Build history of the part. All positions in model axes, mm. A direction names the side the tool comes from. Give positions to 0.01 mm unless a question says otherwise; leave off trailing zeros. Order: outer loops, then holes, each group sorted by start corner. A loop starts at its lowest first (then second) coordinate and runs counter-clockwise, first axis right, second up. Notation, with made-up numbers: (84.25, 46) - (101.25, 46) arc R24 ccw to (101.25, 57) - close; hole circle Ø10 at (17.25, 60). An arc over 180 degrees is marked (long way). Use a Markdown table: item, result. Add a question column.
(1) Slice it at B-B (z = 94). Write the cut outline in (x, y).
(2) Flat gauge pin, fed straight in: pin 1 (2.5 mm diameter, centred on y = 0, z = 243.79, fed in from -X). Where does the tip first touch, or does it go through?
(3) Mould opens along X. For faces 1 (the face through (0, -7, 253)), 2 (the face through (-7.5, 0, 125)), 3 (the face through (7.5, 0, 125)), 4 (the face through (0.09, -6.74, 1.95)) say: +X half, -X half, draft (parallel to the pull), parting line (faces both ways), or undercut.
(4) Wall check: line 1 (X direction, y = 2.5, z = 176.5); line 2 (X direction, y = -6.95, z = 112). Give the ranges that are in metal, low to high.
(5) Slice it at A-A (z = 53). Write the cut outline in (x, y), then the cut area to 3 significant figures.
(6) Which spindle directions (+Z, -Z, +X, -X, +Y, -Y) get a long thin tool onto all of the face, cutting with end or side? Do faces 5 (the face through (-6.74, 0.09, 55.05)), 6 (the face through (6, 0, 125)). Say none if no direction does.
from build123d import *

# Parameters (mm, degrees)
SKETCH_1_W          = 15
SKETCH_1_H          = 15
SKETCH_1_W_2        = 12
SKETCH_1_H_2        = 12
EXTRUDE_1_DEPTH     = 375
SKETCH_3_R          = 2.05
CUT_EXTRUDE_2_DEPTH = 21
SKETCH_4_R          = 2.05
CUT_EXTRUDE_3_DEPTH = 25
SKETCH_6_R          = 2
CUT_EXTRUDE_5_DEPTH = 75
SKETCH_7_R          = 2
CUT_EXTRUDE_6_DEPTH = 376.374812687
SKETCH_8_W          = 122
SKETCH_8_H          = 15
CUT_EXTRUDE_7_DEPTH = 376.374812687
SKETCH_9_R          = 1.5
CUT_EXTRUDE_8_DEPTH = 254.55522081


with BuildPart() as part:
    # 草图1 → 凸台-拉伸1 (new body)
    with BuildSketch(Plane.XY):
        Rectangle(SKETCH_1_W, SKETCH_1_H)
        Rectangle(SKETCH_1_W_2, SKETCH_1_H_2, mode=Mode.SUBTRACT)
    extrude(amount=EXTRUDE_1_DEPTH)

    # 草图3 → 切除-拉伸2 (cut)
    with BuildSketch(Plane(origin=(0, 7.5, 0), x_dir=(1, 0, 0), z_dir=(0, 1, 0))):
        with Locations(Location((0, -4, 0), (0, 0, 270))):
            Circle(SKETCH_3_R)
        with Locations(Location((0, -12, 0), (0, 0, 270))):
            Circle(SKETCH_3_R)
    extrude(amount=-CUT_EXTRUDE_2_DEPTH, mode=Mode.SUBTRACT)

    # 草图4 → 切除-拉伸3 (cut)
    with BuildSketch(Plane(origin=(7.5, 0, 0), x_dir=(0, 0, -1), z_dir=(1, 0, 0))):
        with Locations((-23, 0)):
            Circle(SKETCH_4_R)
        with Locations((-53, 0)):
            Circle(SKETCH_4_R)
    extrude(amount=-CUT_EXTRUDE_3_DEPTH, mode=Mode.SUBTRACT)

    # 草图6 → 切除-拉伸5 (cut)
    with BuildSketch(Plane(origin=(0, 7.5, 0), x_dir=(1, 0, 0), z_dir=(0, 1, 0))):
        with Locations(Location((0, -335, 0), (0, 0, 270))):
            Circle(SKETCH_6_R)
        with Locations(Location((0, -350, 0), (0, 0, 270))):
            Circle(SKETCH_6_R)
    extrude(amount=-CUT_EXTRUDE_5_DEPTH, mode=Mode.SUBTRACT)

    # 草图7 → 切除-拉伸6 (cut, through all)
    with BuildSketch(Plane(origin=(7.5, 0, 0), x_dir=(0, 0, -1), z_dir=(1, 0, 0))):
        with Locations((-253.786796565, 0)):
            Circle(SKETCH_7_R)
        with Locations((-243.786796565, 0)):
            Circle(SKETCH_7_R)
    extrude(amount=-CUT_EXTRUDE_6_DEPTH, mode=Mode.SUBTRACT)

    # 草图8 → 切除-拉伸7 (cut, through all)
    with BuildSketch(Plane(origin=(7.5, 0, 0), x_dir=(0, 0, -1), z_dir=(1, 0, 0))):
        with Locations((-314, 0)):
            Rectangle(SKETCH_8_W, SKETCH_8_H)
    extrude(amount=-CUT_EXTRUDE_7_DEPTH, mode=Mode.SUBTRACT)

    # 草图9 → 切除-拉伸8 (cut, through all)
    with BuildSketch(Plane(origin=(0, 7.5, 0), x_dir=(1, 0, 0), z_dir=(0, 1, 0))):
        with Locations(Location((0, -218, 0), (0, 0, 270))):
            Circle(SKETCH_9_R)
        with Locations(Location((0, -208, 0), (0, 0, 270))):
            Circle(SKETCH_9_R)
        with Locations(Location((0, -170, 0), (0, 0, 270))):
            Circle(SKETCH_9_R)
        with Locations(Location((0, -160, 0), (0, 0, 270))):
            Circle(SKETCH_9_R)
        with Locations(Location((0, -122, 0), (0, 0, 270))):
            Circle(SKETCH_9_R)
        with Locations(Location((0, -112, 0), (0, 0, 270))):
            Circle(SKETCH_9_R)
        with Locations(Location((0, -74, 0), (0, 0, 270))):
            Circle(SKETCH_9_R)
        with Locations(Location((0, -64, 0), (0, 0, 270))):
            Circle(SKETCH_9_R)
    extrude(amount=-CUT_EXTRUDE_8_DEPTH, mode=Mode.SUBTRACT)


solid = part.part
Solution:
| question | item | result |
|---|---|---|
| 1 | outline | (-7.5, -7.5) - (7.5, -7.5) - (7.5, 7.5) - (-7.5, 7.5) - close; hole (-6, -6) - (6, -6) - (6, 6) - (-6, 6) - close |
| 2 | pin 1 | through |
| 3 | face 1 | draft |
| 3 | face 2 | -X half |
| 3 | face 3 | +X half |
| 3 | face 4 | undercut |
| 4 | line 1 | -7.5 to -6, 6 to 7.5 |
| 4 | line 2 | -7.5 to -1.5, 1.5 to 7.5 |
| 5 | outline | (-7.5, -7.5) - (7.5, -7.5) - (7.5, -2.05) - (6, -2.05) - (6, -6) - (-6, -6) - (-6, -2.05) - (-7.5, -2.05) - close; (-7.5, 2.05) - (-6, 2.05) - (-6, 6) - (6, 6) - (6, 2.05) - (7.5, 2.05) - (7.5, 7.5) - (-7.5, 7.5) - close |
| 5 | area | 68.7 mm2 |
| 6 | face 5 | +X, -X |
| 6 | face 6 | +Z, -Z |
